Geometry: final body of the model. Coordinates: model frame, mm. A direction names the side the tool comes from. Give positions to 0.01 mm unless a question says otherwise; leave off trailing zeros. Loops run counter-clockwise (first coordinate to the right, second up) from the corner with the lowest first, then second, coordinate; pieces in that order, holes last. Notation, with made-up numbers: (30.25, 30.5) -> (72.25, 30.5) arc R22 cw to (72.25, 39.5) -> close; hole circle Ø1 at (20, 11.5). An arc over 180 degrees is marked (long way). Answer in a Markdown table with one row per item. Add a question column.
1) Section query C-C (z = -17.5). Return the cut outline in (x, y).
2) Section query D-D (y = -15.5). Return the cut outline in (x, z).
3) Section query B-B (y = 7). Return the cut outline in (x, z), plus the area to 3 significant figures.
4) Draft query along X for faces 5 (the flat face through (-27.05, 31, -21)), 6 (the flat face through (-20, 15.15, -21)), 7 (the flat face through (22, -21.5, -21)). Return one class per face: +X half, -X half, draft (parallel to the pull), parting line (faces both ways), or undercut.
5) Line query: line 1 (Y direction, x = -20, z = -3); line 2 (X direction, y = 15, z = -39); line 3 (Y direction, x = 39, z = -30). Output: solid intervals per line, ascending. Write a range as from..to.
6) Section query A-A (x = -23). Return the cut outline in (y, z).
7) Access query for faces 1 (the flat face through (-20, 40.55, -21)), 2 (the flat face through (47, 5, -33)), 3 (the flat face through (-14, 44, -21)), 4 (the flat face through (43.65, -9, -36)). Directions: +Z, -Z, +X, -X, +Y, -Y. A direction counts if a zero-diameter tool reaches every point of the face in a straight line with its end or side. Return the directions, or none.
8) First-contact query: P1, Ø5, axis at y = 25.5, z = -21, coming from the +X side; P2, Ø3, axis at x = 47.5, z = -19.5, coming from the +Y side; P3, Ø1.9, axis at y = -15.21, z = -36.71, coming from the -X side; P4, Ø1.9, axis at x = 46.5, y = 12.5, coming from the +Z side. Flat tips, straight axial feed; report the tip coordinate or a pass-through.
```python
from build123d import *

# Parameters (mm, degrees)
BOSS_EXTRUDE1_DEPTH     = 43
SKETCH2_W               = 33
SKETCH2_H               = 6.35
SKETCH2_H_2             = 10
SKETCH2_R               = 1.5
SKETCH2_W_2             = 10
BOSS_EXTRUDE2_DEPTH     = 6.35
CUT_EXTRUDE1_DEPTH      = 85.993720356
CUT_EXTRUDE1_DEPTH_BACK = 12.7
SKETCH3_R               = 1.5875


with BuildPart() as part:
    # Sketch1 → Boss-Extrude1 (new body)
    with BuildSketch(Plane.XY):
        Polygon((-6.35, -27.85), (-6.35, 15.15), (-33.4, 15.15), (-33.4, 46.9), (-14, 46.9), (-14, 40.55), (-27.05, 40.55), (-27.05, 21.5), (0, 21.5), (0, -21.5), (43.65, -21.5), (43.65, -27.85), align=None)
    extrude(amount=-BOSS_EXTRUDE1_DEPTH)

    # Sketch2 → Boss-Extrude2 (add)
    # profile 1 of 4: a face of its own
    with BuildSketch(Plane(origin=(43.65, 0, 0), x_dir=(0, 0, -1), z_dir=(1, 0, 0))):
        with Locations((16.5, -24.675)):
            Rectangle(SKETCH2_W, SKETCH2_H)
    # profile 2 of 4: a face of its own
    with BuildSketch(Plane(origin=(43.65, 0, 0), x_dir=(0, 0, -1), z_dir=(1, 0, 0))):
        with Locations((16.5, -16.5)):
            Rectangle(SKETCH2_W, SKETCH2_H_2)
        with Locations((6.294174233, -15.205825767)):
            Circle(SKETCH2_R, mode=Mode.SUBTRACT)
    # profile 3 of 4: a face of its own
    with BuildSketch(Plane(origin=(43.65, 0, 0), x_dir=(0, 0, -1), z_dir=(1, 0, 0))):
        with Locations((38, -24.675)):
            Rectangle(SKETCH2_W_2, SKETCH2_H)
    # profile 4 of 4: a face of its own
    with BuildSketch(Plane(origin=(43.65, 0, 0), x_dir=(0, 0, -1), z_dir=(1, 0, 0))):
        Polygon((33, -11.5), (33, -21.5), (43, -21.5), (43, 21.5), (33, 21.5), align=None)
        with Locations((36.705825767, -15.205825767)):
            Circle(SKETCH2_R, mode=Mode.SUBTRACT)
        with Locations((36.705825767, 15.205825767)):
            Circle(SKETCH2_R, mode=Mode.SUBTRACT)
    extrude(amount=BOSS_EXTRUDE2_DEPTH)

    # Sketch3 → Cut-Extrude1 (cut, two sides: drawn at the far end of the back side and taken through both)
    with BuildSketch(Plane(origin=(-6.35, 0, 0), x_dir=(0, 0, -1), z_dir=(1, 0, 0)).offset(-CUT_EXTRUDE1_DEPTH_BACK)):
        with Locations(Location((6.294174233, -15.205825767, 0), (0, 0, 270))):
            Circle(SKETCH3_R)
        with Locations(Location((6.294174233, 15.205825767, 0), (0, 0, 270))):
            Circle(SKETCH3_R)
        with Locations(Location((36.705825767, 15.205825767, 0), (0, 0, 270))):
            Circle(SKETCH3_R)
        with Locations(Location((36.705825767, -15.205825767, 0), (0, 0, 270))):
            Circle(SKETCH3_R)
    extrude(amount=CUT_EXTRUDE1_DEPTH + CUT_EXTRUDE1_DEPTH_BACK, mode=Mode.SUBTRACT)


solid = part.part
```
Evaluation:
| question | item | result |
|---|---|---|
| 1 | outline | (-33.4, 15.15) -> (-6.35, 15.15) -> (-6.35, -27.85) -> (50, -27.85) -> (50, -11.5) -> (43.65, -11.5) -> (43.65, -21.5) -> (0, -21.5) -> (0, 21.5) -> (-27.05, 21.5) -> (-27.05, 40.55) -> (-14, 40.55) -> (-14, 46.9) -> (-33.4, 46.9) -> close |
| 2 | outline | (-6.35, -43) -> (0, -43) -> (0, -38.27) -> (-6.35, -38.27) -> close; (-6.35, -35.15) -> (0, -35.15) -> (0, -7.85) -> (-6.35, -7.85) -> close; (-6.35, -4.73) -> (0, -4.73) -> (0, 0) -> (-6.35, 0) -> close; (43.65, -43) -> (50, -43) -> (50, -38.27) -> (43.65, -38.27) -> close; (43.65, -35.15) -> (50, -35.15) -> (50, -7.85) -> (43.65, -7.85) -> close; (43.65, -4.73) -> (50, -4.73) -> (50, 0) -> (43.65, 0) -> close |
| 3 | outline | (-6.35, -43) -> (0, -43) -> (0, 0) -> (-6.35, 0) -> close; (43.65, -43) -> (50, -43) -> (50, -33) -> (43.65, -33) -> close |
| 3 | area | 337 mm² |
| 4 | face 5 | +X half |
| 4 | face 6 | draft |
| 4 | face 7 | undercut |
| 5 | line 1 | 15.15..21.5, 40.55..46.9 |
| 5 | line 2 | -6.35..0, 43.65..50 |
| 5 | line 3 | -27.85..-21.5 |
| 6 | outline | (15.15, -43) -> (21.5, -43) -> (21.5, 0) -> (15.15, 0) -> close; (40.55, -43) -> (46.9, -43) -> (46.9, 0) -> (40.55, 0) -> close |
| 7 | face 1 | +Z, -Z, +X |
| 7 | face 2 | +Z, +X, +Y |
| 7 | face 3 | +Z, -Z, +X, +Y |
| 7 | face 4 | +Z, -Z, +Y |
| 8 | P1 | x = -27.05 |
| 8 | P2 | y = -11.5 |
| 8 | P3 | through |
| 8 | P4 | z = -33 |
